```python
from build123d import *

# Parameters (mm, degrees)
SKETCH3_W           = 25.4
SKETCH3_H           = 25.4
SKETCH3_W_2         = 19.304
SKETCH3_H_2         = 19.304
BOSS_EXTRUDE1_DEPTH = 500
FILLET1_R           = 2.5
FILLET2_R           = 1
CUT_EXTRUDE1_DEPTH  = 501.805800685


with BuildPart() as part:
    # Sketch3 → Boss-Extrude1 (new body)
    with BuildSketch(Plane(origin=(0, 0, 0), x_dir=(0, 0, -1), z_dir=(1, 0, 0))):
        Rectangle(SKETCH3_W, SKETCH3_H)
        Rectangle(SKETCH3_W_2, SKETCH3_H_2, mode=Mode.SUBTRACT)
    extrude(amount=-BOSS_EXTRUDE1_DEPTH)

    # Fillet1
    fillet1_edges = [part.edges().sort_by_distance(p)[0] for p in [
        (-250, -12.7, -12.7),
        (-250, -12.7, 12.7),
        (-250, 12.7, 12.7),
        (-250, 12.7, -12.7),
    ]]
    fillet(fillet1_edges, radius=FILLET1_R)

    # Fillet2
    fillet2_edges = [part.edges().sort_by_distance(p)[0] for p in [
        (-250, 9.652, -9.652),
        (-250, -9.652, -9.652),
        (-250, -9.652, 9.652),
        (-250, 9.652, 9.652),
    ]]
    fillet(fillet2_edges, radius=FILLET2_R)

    # Sketch4 → Cut-Extrude1 (cut, through all)
    with BuildSketch(Plane.XY.offset(12.7)):
        Polygon((-482.303319661, -10.2), (-500, -4.45), (-500, -10.2), align=None)
        Polygon((-474.609110818, -12.7), (-482.303319661, -10.2), (-500, -10.2), (-500, -12.7), align=None)
    extrude(amount=-CUT_EXTRUDE1_DEPTH, mode=Mode.SUBTRACT)


solid = part.part
```
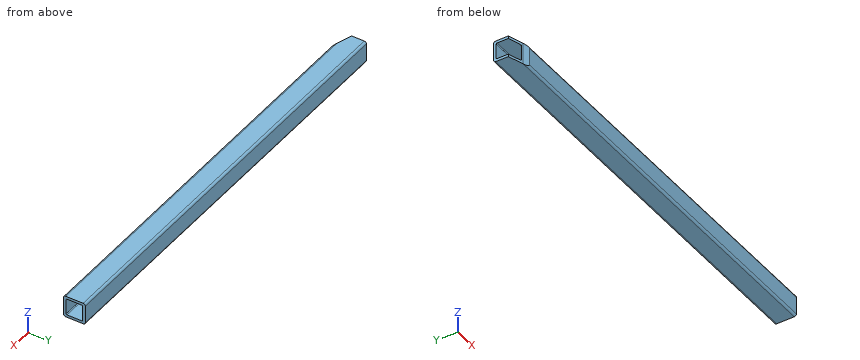
The model under review builds one solid part; all positions refer to its coordinate system, in mm. Round coordinates to 2 decimals unless told otherwise and drop trailing zeros. Loops run counter-clockwise (first coordinate to the right, second up) from the corner with the lowest first, then second, coordinate; pieces in that order, holes last. Notation, with made-up numbers: (57, 27.25) -> (84, 27.25) arc R23 ccw to (84, 51.25) -> close; hole circle Ø2 at (51, -4). An arc over 180 degrees is marked (long way). Answer as a JSON object with one key per item and string values. Group by question number.
1) We need section A-A on y = 0. Write out the cut boundary in (x, z), then the cut area to 3 significant figures.
2) For pin 1 Ø2 at (y, z) = (1.5, -7) entering from +X, flat-tipped, find the tip position at first contact; note if it passes through.
3) We need section C-C on x = -34. Write out the cut boundary in (y, z).
4) We need section B-B on z = 3.75. Write out the cut boundary in (x, y).
5) For line 1 (Z direction, x = -327, y = 8); line 2 (Y direction, x = -406.5, z = -9), list the stretches that pass through material, from the lowest coordinate up. Write a range as [from, to].
Result set:
{
 "1": {"outline": "(-500, -12.7) -> (0, -12.7) -> (0, -9.65) -> (-500, -9.65) -> close; (-500, 9.65) -> (0, 9.65) -> (0, 12.7) -> (-500, 12.7) -> close", "area": "3,050 mm²"},
 "2": {"pin 1": "through"},
 "3": {"outline": "(-12.7, -10.2) arc R2.5 ccw to (-10.2, -12.7) -> (10.2, -12.7) arc R2.5 ccw to (12.7, -10.2) -> (12.7, 10.2) arc R2.5 ccw to (10.2, 12.7) -> (-10.2, 12.7) arc R2.5 ccw to (-12.7, 10.2) -> close; hole (-9.65, -8.65) arc R1 ccw to (-8.65, -9.65) -> (8.65, -9.65) arc R1 ccw to (9.65, -8.65) -> (9.65, 8.65) arc R1 ccw to (8.65, 9.65) -> (-8.65, 9.65) arc R1 ccw to (-9.65, 8.65) -> close"},
 "4": {"outline": "(-500, 9.65) -> (0, 9.65) -> (0, 12.7) -> (-500, 12.7) -> close; (-483.99, -9.65) -> (-474.61, -12.7) -> (0, -12.7) -> (0, -9.65) -> close"},
 "5": {"line 1": "[-12.7, -9.65], [9.65, 12.7]", "line 2": "[-12.7, -9.59], [9.59, 12.7]"}
}
